The model under review builds one solid part; all positions refer to its coordinate system, in mm. A direction names the side the tool comes from. Round coordinates to 2 decimals unless told otherwise and drop trailing zeros. Order: outer loops, then holes, each group sorted by start corner. A loop starts at its lowest first (then second) coordinate and runs counter-clockwise, first axis right, second up. Notation, with made-up numbers: M 36.25,27.25 L 81.25,27.25 A16 ccw 81.25,49.25 Z; hole C 9.25,76 d11. An arc over 180 degrees is marked long. Answer as a JSON object with one key per item and string values. Group by question number.
1) Insertion check: pin 1 Ø5 at (x, z) = (12.5, 66.5) entering from -Y; pin 2 Ø4 at (y, z) = (-5, 43.5) entering from +X; pin 3 Ø2 at (y, z) = (22.5, 50.5) entering from -X. Each pin has a flat end and moves straight along its axis. Give the tip position at first contact, or say it passes through.
2) To check wall thickness, follow line 1 (X direction, y = 15.5, z = 155); line 2 (Z direction, x = -35.5, y = 12.5). State the ranges of each line that lie inside material, in increasing order.
3) Consider section A-A, the plane x = -9.5. Write out the cut boundary in (y, z), then the cut area to 3 significant figures.
4) For faces 1 (the flat face through (-35, 0, 110)), 2 (the cylindrical face through (-39, -38, 0)), 3 (the flat face through (0, -35, 110)), 4 (the flat face through (35, 0, 110)), 5 (the flat face through (0, 35, 110)), list the 3-axis set-ups (+Z, -Z, +X, -X, +Y, -Y) from which the entire face can be reached by the end or side of a thin tool; tool diameter is ignored.
5) Consider section C-C, the plane z = 48.5. Write out the cut boundary in (x, y), then the cut area to 3 significant figures.
```python
from build123d import *

# Parameters (mm, degrees)
F0_W     = 80
F0_H     = 80
F1_DEPTH = 40
F2_R     = 5
F3_DEPTH = 80.001


# Not quite as in the source:
# - a pattern or mirror of a feature is missing from the dataset's text; its kind, count and spacing are read off the source's solid


with BuildPart() as f1:
    # F0 (on Top) → F1 (new body, symmetric)
    with BuildSketch(Plane.XY):
        Rectangle(F0_W, F0_H)
    extrude(amount=F1_DEPTH, both=True)

    # F2
    f2_edges = [f1.edges().sort_by_distance(p)[0] for p in [
        (0, 40, 40),
        (-40, 0, 40),
        (40, 0, 40),
        (0, -40, 40),
        (40, 40, 0),
        (40, -40, 0),
        (40, 0, -40),
        (-40, 40, 0),
        (-40, 0, -40),
        (-40, -40, 0),
        (0, -40, -40),
        (0, 40, -40),
    ]]
    fillet(f2_edges, radius=F2_R)

    # F3 (add, through all): faces of the model
    f3_faces = [f1.faces().sort_by_distance(p)[0] for p in [
        (0, 0, -40),
        (0, 0, 40),
    ]]
    f3 = extrude(f3_faces, amount=-F3_DEPTH, dir=(0, 0, -1))

    # F3_copies: F3 across plane
    add(f3.mirror(Plane.XY.offset(69.287032)))


solid = f1.part
```
Results list:
{
 "1": {"pin 1": "y = -35", "pin 2": "x = 35", "pin 3": "x = -35"},
 "2": {"line 1": "-35 to 35", "line 2": "-39.97 to 39.97"},
 "3": {"outline": "M -40,-35 A5 ccw -35,-40 L 35,-40 A5 ccw 40,-35 L 40,35 A5 ccw 35,40 L 35,178.57 L -35,178.57 L -35,40 A5 ccw -40,35 Z", "area": "16,100 mm^2"},
 "4": {"face 1": "+Z, -X, +Y, -Y", "face 2": "+Z, -Z, -X, -Y", "face 3": "+Z, +X, -X, -Y", "face 4": "+Z, +X, +Y, -Y", "face 5": "+Z, +X, -X, +Y"},
 "5": {"outline": "M -35,-35 L 35,-35 L 35,35 L -35,35 Z", "area": "4,900 mm^2"}
}
